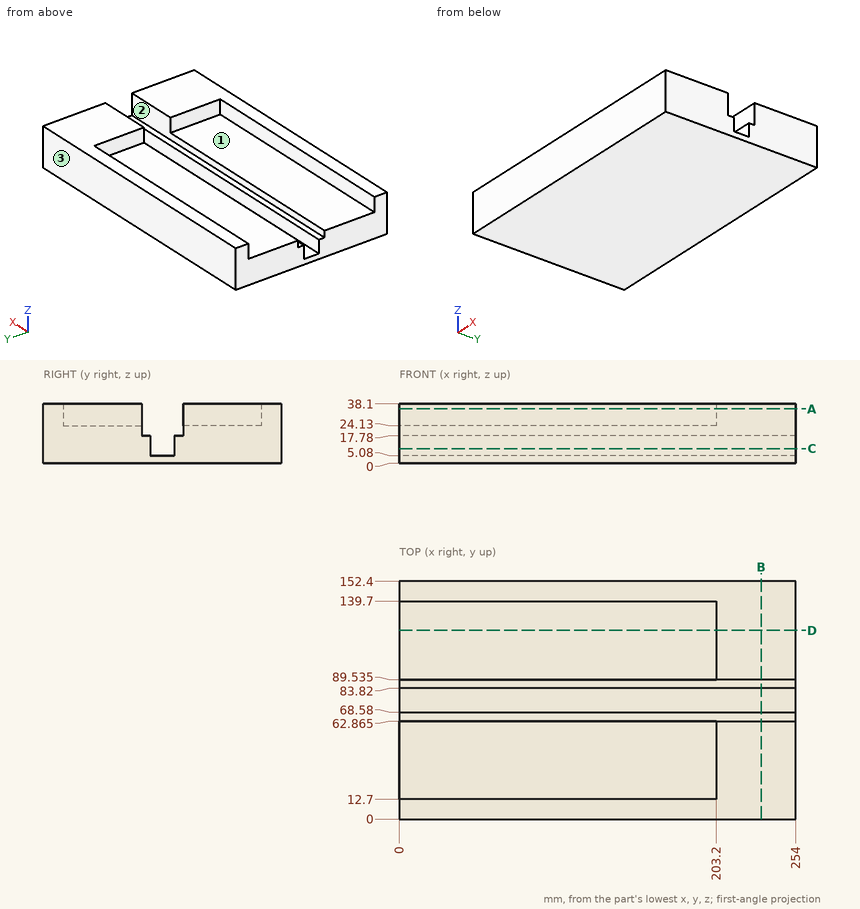
Drawing for the job (mm, zero at the part's lowest x, y, z). A direction names the side the tool comes from. Round coordinates to 2 decimals unless told otherwise and drop trailing zeros. Loops run counter-clockwise (first coordinate to the right, second up) from the corner with the lowest first, then second, coordinate; pieces in that order, holes last. Notation, with made-up numbers: (66.25, 4) -> (76.25, 4) arc R25 cw to (76.25, 31) -> close; hole circle Ø3 at (-9.5, -7). An arc over 180 degrees is marked (long way). Answer in a Markdown table with one row per item.
Item 1: Saw through at B-B (x = 232). Write the cut outline in (y, z) (3 decimals).
Answers below:
| item | result |
|---|---|
| outline | (0, 0) -> (152.4, 0) -> (152.4, 38.1) -> (89.535, 38.1) -> (89.535, 17.78) -> (83.82, 17.78) -> (83.82, 5.08) -> (68.58, 5.08) -> (68.58, 17.78) -> (62.865, 17.78) -> (62.865, 38.1) -> (0, 38.1) -> close |
Item 2: Which spindle directions (+Z, -Z, +X, -X, +Y, -Y) get a long thin tool onto all of the face, cutting with end or side? Do the marked faces 1, 2 and 3. Say none if no direction does.
Answers below:
| item | result |
|---|---|
| face 1 | +Z, -X |
| face 2 | +Z, +X, -X |
| face 3 | +Z, -Z, +X, -X, +Y |
Item 3: Saw through at C-C (z = 9.5). Write the cut outline in (x, y), and give its area (3 significant figures).
Answers below:
| item | result |
|---|---|
| outline | (0, 0) -> (254, 0) -> (254, 68.58) -> (0, 68.58) -> close; (0, 83.82) -> (254, 83.82) -> (254, 152.4) -> (0, 152.4) -> close |
| area | 34,800 mm² |
Item 4: Drill centre lines: L1, parallel to Y at x = 58.5, z = 26.5; L2, parallel to Y at x = 49.5, z = 16.5; L3, parallel to Z at x = 167, y = 126. Where is each one in solid material? Low to high. Write a range as [from, to].
Answers below:
| item | result |
|---|---|
| L1 | y = [0, 12.7], [139.7, 152.4] |
| L2 | y = [0, 68.58], [83.82, 152.4] |
| L3 | z = [0, 24.13] |
Item 5: Saw through at A-A (z = 35). Write the cut outline in (x, y) (3 decimals), and give its area (3 significant figures).
Answers below:
| item | result |
|---|---|
| outline | (0, 0) -> (254, 0) -> (254, 62.865) -> (203.2, 62.865) -> (203.2, 12.7) -> (0, 12.7) -> close; (0, 139.7) -> (203.2, 139.7) -> (203.2, 89.535) -> (254, 89.535) -> (254, 152.4) -> (0, 152.4) -> close |
| area | 11,500 mm² |
Item 6: Saw through at D-D (y = 121). Write the cut outline in (x, z).
Answers below:
| item | result |
|---|---|
| outline | (0, 0) -> (254, 0) -> (254, 38.1) -> (203.2, 38.1) -> (203.2, 24.13) -> (0, 24.13) -> close |
Item 7: Pin check, flat tips, straight feed: pin 1 (2 mm diameter, centred on x = 76.5, y = 39.5, fed in from +Z); pin 2 (14 mm diameter, centred on x = 108, z = 9.5, fed in from -Y); pin 3 (3 mm diameter, centred on x = 110.5, y = 64.5, fed in from +Z); pin 4 (15.5 mm diameter, centred on y = 108, z = 32.5, fed in from -X). Stop position of each tip, or through.
Answers below:
| item | result |
|---|---|
| pin 1 | stops at z = 24.13 |
| pin 2 | stops at y = 0 |
| pin 3 | stops at z = 17.78 |
| pin 4 | stops at x = 203.2 |
